```python
from build123d import *

# Parameters (mm, degrees)
SKETCH012_R     = 1.1
PAD007_DEPTH    = 3
SKETCH013_R     = 4
SKETCH013_R_2   = 1.1
PAD008_DEPTH    = 1
SKETCH014_R     = 0.95
PAD009_DEPTH    = 4.5
SKETCH016_R     = 2.35
POCKET003_DEPTH = 2.5
FILLET002_R     = 0.9


with BuildPart() as part:
    # Sketch012 → Pad007 (new body)
    with BuildSketch(Plane(origin=(26.5, -4.5, -11), x_dir=(1, 0, 0), z_dir=(0, 0, 1))):
        with BuildLine():
            Line((-11.827489, -0.965926), (-1.202823, -3.814868))
            ThreePointArc((-1.202823, -3.814868), (4, 0), (-1.202823, 3.814868))
            Line((-11.827489, 0.965926), (-1.202823, 3.814868))
            ThreePointArc((-11.827489, 0.965926), (-12.56867, 0), (-11.827489, -0.965926))
        make_face()
        Circle(SKETCH012_R, mode=Mode.SUBTRACT)
    extrude(amount=PAD007_DEPTH)

    # Sketch013 → Pad008 (new body)
    with BuildSketch(Plane(origin=(26.5, -4.5, -11), x_dir=(1, 0, 0), z_dir=(0, 0, -1))):
        Circle(SKETCH013_R)
        Circle(SKETCH013_R_2, mode=Mode.SUBTRACT)
    extrude(amount=PAD008_DEPTH)

    # Sketch014 → Pad009 (new body)
    with BuildSketch(Plane(origin=(26.5, -4.5, -11), x_dir=(1, 0, 0), z_dir=(0, 0, -1))):
        with Locations((-11.56867, 0)):
            Circle(SKETCH014_R)
    extrude(amount=PAD009_DEPTH)

    # Sketch016 → Pocket003 (cut)
    with BuildSketch(Plane(origin=(26.5, -4.5, -8), x_dir=(1, 0, 0), z_dir=(0, 0, 1))):
        Circle(SKETCH016_R)
    extrude(amount=-POCKET003_DEPTH, mode=Mode.SUBTRACT)

    # Fillet002
    fillet002_edges = [part.edges().sort_by_distance(p)[0] for p in [
        (13.98133, -4.5, -15.5),
    ]]
    fillet(fillet002_edges, radius=FILLET002_R)


solid = part.part
```
Here's how the part is built. I have some questions about the finished solid (model axes, mm). A direction names the side the tool comes from. Give positions to 0.01 mm unless a question says otherwise; leave off trailing zeros. Order: outer loops, then holes, each group sorted by start corner. A loop starts at its lowest first (then second) coordinate and runs counter-clockwise, first axis right, second up. Notation, with made-up numbers: (48.5, 30) - (72.5, 30) arc R27 ccw to (72.5, 69) - close; hole circle Ø8 at (50.5, 83.5). An arc over 180 degrees is marked (long way). Answer as a JSON object with one key per item and string values. Group by question number.
Item 1: If we section it at D-D on x = 23: Please give me the cut outline in (y, z).
Item 2: Which directions (+Z, -Z, +X, -X, +Y, -Y) give clear straight access to the entire face, cutting with the end or side of a thin tool? Please do faces 5 (the cylindrical face through (15.81, -4.14, -12.77)), 6 (the cylindrical face through (24.152, -4.397, -9.232)), 7 (the flat face through (27.33, -5.44, -12)).
Item 3: Please list where these lines run through material, in increasing order: probe 1 along Y at (x, z) = (26.5, -10.95); probe 2 along X at (y, z) = (-4.5, -11.5); probe 3 along Y at (x, z) = (26.5, -9.55).
Item 4: If we section it at A-A on x = 26.5: Please give me the cut outline in (y, z), and give its area (4 significant figures).
Item 5: If we mould it in two halves opening along Y, with no side actions, what happens to faces 1 (the flat face through (27, -6, -10.5)), 2 (the cylindrical face through (13.93, -4.48, -9.52)), 3 (the cylindrical face through (25.4, -4.5, -11.2)), 4 (the flat face through (22, -4, -8))? For each: pulls with the +Y half, pulls with the -Y half, needs draft (parallel to the pull), parting line crosses it, or undercut.
Item 6: For P1, Ø3.5, axis at x = 26.5, y = -4.5, coming from the +Z side; P2, Ø1, axis at x = 19.5, y = -2, coming from the -Z side; P3, Ø3, axis at x = 26.5, y = -4.5, coming from the -Z side, each with a flat end and sliding along its axis, tell me the tip position at first contact or that it passes through.
Item 7: If we section it at C-C on z = -12.75: Please give me the cut outline in (x, y), and give its area (3 significant figures).
Item 8: If we section it at B-B on y = -1.5: Please give me the cut outline in (x, z), and give its area (3 significant figures).
Result set:
{
 "1": {"outline": "(-7.7, -11) - (-6.44, -11) - (-6.44, -12) - (-2.56, -12) - (-2.56, -11) - (-1.3, -11) - (-1.3, -8) - (-7.7, -8) - close"},
 "2": {"face 5": "-Z", "face 6": "+Z", "face 7": "-Z, +X, +Y, -Y"},
 "3": {"probe 1": "-8.5 to -5.6, -3.4 to -0.5", "probe 2": "13.98 to 15.88, 22.5 to 25.4, 27.6 to 30.5", "probe 3": "-8.5 to -6.85, -2.15 to -0.5"},
 "4": {"outline": "(-8.5, -12) - (-5.6, -12) - (-5.6, -10.5) - (-6.85, -10.5) - (-6.85, -8) - (-8.5, -8) - close; (-3.4, -12) - (-0.5, -12) - (-0.5, -8) - (-2.15, -8) - (-2.15, -10.5) - (-3.4, -10.5) - close", "area": "16.95 mm²"},
 "5": {"face 1": "undercut", "face 2": "parting line crosses it", "face 3": "undercut", "face 4": "needs draft"},
 "6": {"P1": "z = -10.5", "P2": "z = -11", "P3": "z = -12"},
 "7": {"outline": "circle Ø1.9 at (14.93, -4.5)", "area": "2.84 mm²"},
 "8": {"outline": "(22.26, -11) - (23.85, -11) - (23.85, -12) - (29.15, -12) - (29.15, -8) - (22.26, -8) - close", "area": "26.0 mm²"}
}
